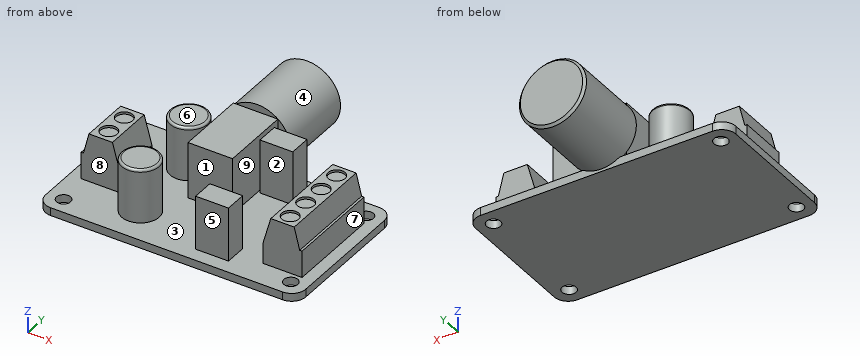
Autodesk Inventor part; units mm, degrees
ref_plane "YZ Plane" through (0, 0, 0) normal (1, 0, 0) x (0, 1, 0)
ref_plane "XZ Plane" through (0, 0, 0) normal (0, 1, 0) x (-1, 0, 0)
ref_plane "XY Plane" through (0, 0, 0) normal (0, 0, 1) x (1, 0, 0)
sketch "Board" plane through (0, 0, 0) normal (0, 0, 1) x (1, 0, 0)
  line L0 (-27.75, 16) -> (27.75, 16)
  line L1 (27.75, 16) -> (27.75, -16)
  line L2 (27.75, -16) -> (-27.75, -16)
  line L3 (-27.75, -16) -> (-27.75, 16)
  line L4 (-27.75, 16) -> (27.75, -16) construction
  line L5 (27.75, 16) -> (-27.75, -16) construction
  line L6 (-24.25, -12.5) -> (24.25, -12.5) construction
  line L7 (24.25, -12.5) -> (24.25, 12.5) construction
  line L8 (24.25, 12.5) -> (-24.25, 12.5) construction
  line L9 (-24.25, 12.5) -> (-24.25, -12.5) construction
  line L10 (-24.25, -12.5) -> (24.25, 12.5) construction
  line L11 (24.25, -12.5) -> (-24.25, 12.5) construction
  circle A0 centre (24.25, 12.5) radius 1.5
  circle A1 centre (-24.25, 12.5) radius 1.5
  circle A2 centre (24.25, -12.5) radius 1.5
  circle A3 centre (-24.25, -12.5) radius 1.5
  line L12 (-25.75, -14) -> (-22.75, -14) construction
  line L13 (-22.75, -14) -> (-22.75, -11) construction
  line L14 (-22.75, -11) -> (-25.75, -11) construction
  line L15 (-25.75, -11) -> (-25.75, -14) construction
  line L16 (-25.75, -14) -> (-22.75, -11) construction
  line L17 (-22.75, -14) -> (-25.75, -11) construction
  point P0 (0, 0)
  dimension "d0" = 55.5
  dimension "d1" = 32
  dimension "d2" = 3
  dimension "d3" = 2
  dimension "d5" = 2
  dimension "d6" = 48.5
extrude "BoardFeature" add sketch "Board" along normal blind 1.7
fillet "BoardFilletsFeature" radius 3 4 edges at (-27.75, 16, 0.85) (27.75, 16, 0.85) (-27.75, -16, 0.85) (27.75, -16, 0.85)
sketch "PotentiometerHousing" plane through (0, 0, 1.7) normal (0, 0, 1) x (1, 0, 0)
  line L0 (-5.75, 15) -> (3.75, 15)
  line L1 (3.75, 15) -> (3.75, 0)
  line L2 (3.75, 0) -> (-5.75, 0)
  line L3 (-5.75, 0) -> (-5.75, 15)
  line L4 (24.75, 16) -> (-24.75, 16)
  line L5 (-27.75, 13) -> (-27.75, -13)
  point P0 (0, 0)
  dimension "d10" = 1
  dimension "d11" = 22
  dimension "d12" = 15
  dimension "d13" = 9.5
extrude "PotentiometerHousingFeature" add sketch "PotentiometerHousing" along normal blind 12
sketch "IJ63" plane through (0, 0, 1.7) normal (0, 0, 1) x (1, 0, 0)
  line L0 (4.25, 13) -> (11.25, 13)
  line L1 (11.25, 13) -> (11.25, 8.3)
  line L2 (11.25, 8.3) -> (4.25, 8.3)
  line L3 (4.25, 8.3) -> (4.25, 13)
  line L4 (3.75, 15) -> (-5.75, 15)
  line L5 (3.75, 0) -> (3.75, 15)
  line L6 (-38.85, 0) -> (38.85, 0) construction
  line L7 (4.25, -13) -> (11.25, -13)
  line L8 (11.25, -13) -> (11.25, -8.3)
  line L9 (11.25, -8.3) -> (4.25, -8.3)
  line L10 (4.25, -8.3) -> (4.25, -13)
  point P0 (0, 0)
  dimension "d16" = 2
  dimension "d17" = 4.7
  dimension "d18" = 7
  dimension "d19" = 0.5
extrude "IJ63Feature" add sketch "IJ63" along normal blind 11.5
sketch "Capacitors" plane through (0, 0, 1.7) normal (0, 0, 1) x (1, 0, 0)
  line L0 (-38.85, 0) -> (38.85, 0) construction
  circle A0 centre (-10.75, 8) radius 4
  line L1 (0, -22.4) -> (0, 22.4) construction
  line L2 (-5.75, 15) -> (-5.75, 0)
  line L3 (24.75, 16) -> (-24.75, 16)
  circle A1 centre (-10.75, -8) radius 4
  point P0 (0, 0)
  dimension "d22" = 8
  dimension "d23" = 5
  dimension "d24" = 8
extrude "CapacitorsFeature" add sketch "Capacitors" along normal blind 11.5
sketch "TerminalBlocks" plane through (0, 0, 1.7) normal (0, 0, 1) x (1, 0, 0)
  line L0 (-38.85, 0) -> (38.85, 0) construction
  line L1 (25.18, 10.25) -> (16.83, 10.25)
  line L2 (16.83, 10.25) -> (16.83, -10.25)
  line L3 (16.83, -10.25) -> (25.18, -10.25)
  line L4 (25.18, -10.25) -> (25.18, 10.25)
  line L5 (-25.18, 5.25) -> (-16.83, 5.25)
  line L6 (-16.83, 5.25) -> (-16.83, -5.25)
  line L7 (-16.83, -5.25) -> (-25.18, -5.25)
  line L8 (-25.18, -5.25) -> (-25.18, 5.25)
  line L9 (27.75, -13) -> (27.75, 13)
  line L10 (-27.75, 13) -> (-27.75, -13)
  point P0 (0, 0)
  point P1 (25.18, 0)
  point P2 (-16.83, 0)
  dimension "d27" = 8.35
  dimension "d28" = 20.5
  dimension "d29" = 10.5
  dimension "d30" = 2.57
  dimension "d31" = 2.57
extrude "TerminalBlocksFeature" add sketch "TerminalBlocks" along normal blind 10.33
sketch "TerminalBlockProfiles" plane through (16.83, -10.25, 1.7) normal (0, -1, 0) x (1, 0, 0)
  line L0 (8.35, 0) -> (0, 0)
  line L1 (8.35, 0) -> (8.35, 10.33)
  line L2 (0, 10.33) -> (8.35, 10.33)
  line L3 (0, 0) -> (0, 10.33)
  line L4 (-33.66, 0) -> (-42.01, 0)
  line L5 (-33.66, 0) -> (-33.66, 10.33)
  line L6 (-42.01, 10.33) -> (-33.66, 10.33)
  line L7 (-42.01, 0) -> (-42.01, 10.33)
  line L8 (0, 10.33) -> (8.35, 10.33)
  line L9 (1.675, 10.33) -> (0, 4.33)
  line L10 (6.675, 10.33) -> (7.85, 5.72)
  line L11 (7.85, 5.72) -> (8.35, 5.72)
  line L12 (8.35, 0) -> (8.35, 10.33)
  line L13 (-16.83, -4.44) -> (-16.83, 14.74) construction
  line L14 (-35.335, 10.33) -> (-33.66, 4.33)
  line L15 (-40.335, 10.33) -> (-41.51, 5.72)
  line L16 (-41.51, 5.72) -> (-42.01, 5.72)
  line L17 (1.675, 10.33) -> (6.675, 10.33)
  point P0 (-16.83, -1.7)
  point P1 (4.175, 10.33)
  point P2 (6.675, 10.33)
  point P3 (1.675, 10.33)
  point P4 (-33.66, 4.33)
  dimension "d34" = 5
  dimension "d35" = 0.5
  dimension "d36" = 4.33
  dimension "d37" = 5.72
extrude "TerminalBlockProfilesFeature" cut sketch "TerminalBlockProfiles" against normal through all contours L11 L10 L2 L1 | L3 L2 L9 | L14 L6 L5 | L7 L6 L15 L16
sketch "TerminalBlockScrews" plane through (0, 0, 12.03) normal (0, 0, 1) x (1, 0, 0)
  line L0 (18.505, 10.25) -> (18.505, -10.25)
  line L1 (18.505, -10.25) -> (23.505, -10.25)
  line L2 (23.505, -10.25) -> (23.505, 10.25)
  line L3 (23.505, 10.25) -> (18.505, 10.25)
  line L4 (-18.505, -5.25) -> (-18.505, 5.25)
  line L5 (-18.505, 5.25) -> (-23.505, 5.25)
  line L6 (-23.505, 5.25) -> (-23.505, -5.25)
  line L7 (-23.505, -5.25) -> (-18.505, -5.25)
  line L8 (18.505, 0) -> (23.505, 0) construction
  line L9 (18.505, 0) -> (23.505, 10.25) construction
  line L10 (21.005, 5.125) -> (23.505, 5.125) construction
  line L11 (23.505, 5.125) -> (18.505, 10.25) construction
  circle A0 centre (21.005, 7.6875) radius 1.8
  circle A1 centre (21.005, 2.5625) radius 1.8
  circle A2 centre (21.005, -7.6875) radius 1.8
  line L12 (21.005, 7.6875) -> (21.005, -7.6875) construction
  circle A3 centre (21.005, -2.5625) radius 1.8
  line L13 (0, -22.4) -> (0, 22.4) construction
  circle A4 centre (-21.005, 2.5625) radius 1.8
  circle A5 centre (-21.005, -2.5625) radius 1.8
  point P0 (0, 0)
  dimension "d41" = 3.6
  dimension "d42" = 2.5625
  dimension "d43" = 2.5625
extrude "TerminalBlockScrewsFeature" cut sketch "TerminalBlockScrews" against normal blind 0.5 contours A0 | A1 | A2 | A3 | A4 | A5
fillet "FilletsFeature" radius 0.5 2 edges at (-14.75, -8, 13.2) (-14.75, 8, 13.2)
sketch "PotentiometerShaft" plane through (-5.75, 15, 1.7) normal (0, 1, 0) x (1, 0, 0)
  line L0 (0, 0) -> (9.5, 0)
  line L1 (0, 0) -> (0, -12)
  line L2 (9.5, -12) -> (0, -12)
  line L3 (9.5, 0) -> (9.5, -12)
  line L4 (9.5, -12) -> (0, 0) construction
  circle A0 centre (4.75, -6) radius 3
  point P0 (5.75, 1.7)
  dimension "d48" = 6
extrude "PotentiometerShaftFeature" add sketch "PotentiometerShaft" along normal blind 0.5 contours A0
sketch "PotentiometerKnob" plane through (-1, 15.5, 7.7) normal (0, 1, 0) x (1, 0, 0)
  circle A0 centre (0, 0) radius 3
  circle A1 centre (0, 0) radius 3
  circle A2 centre (0, 0) radius 7.15
  point P0 (1, 7.7)
  dimension "d51" = 14.3
extrude "PotentiometerKnobFeature" add sketch "PotentiometerKnob" along normal blind 17 contours A0 | A2
chamfer "PotentiometerKnobChamferFeature" distance 0.5 angle 45 1 edges at (-8.15, 32.5, 7.7)
equation "\"d5\" = d3"
equation "\"d31\" = d30"
equation "\"d43\" = d42"
properties part number "LQ-AMP10W"
Design review of the part built by this model. Coordinates are the model's own, in mm. Face numbers are marked on the shaded views. A direction names the side the tool comes from. Give positions to 0.01 mm unless a question says otherwise; leave off trailing zeros. Write each loop counter-clockwise with the first axis right and the second up, starting at its lowest first coordinate (ties: lowest second). Pieces come first, ordered by that corner, then holes. Notation, with made-up numbers: M 47,-36 L 65,-36 A24 cw 65,-1 Z; hole C -24.5,-14.5 d7. An arc over 180 degrees is marked long. Answer as a JSON object with one key per item and string values. Group by question number.
1) We need section B-B (y = 21). Give the boundary of the cut face in (x, z).
2) Mouldability with a two-part tool opening along Y and no side actions: class the marked faces 1, 2, 3 and 4 as released by +Y, released by -Y, zero draft, split by the parting line, or undercut.
3) We need section A-A (x = 7). Give the boundary of the cut face in (y, z).
4) We need section C-C (x = 13.5). Give the boundary of the cut face in (y, z).
5) Clearance check with flat-ended pins moving along their axes: pin 1 Ø2.5 at (x, z) = (21, 9) entering from -Y; pin 2 Ø4 at (x, y) = (-21, -2.56) entering from +Z; pin 3 Ø8 at (x, y) = (-16.5, 4.5) entering from +Z; pin 4 Ø1.8 at (x, y) = (-24.25, -12.5) entering from +Z. State where each tip first meets the part, or that it passes through.
6) For line 1 along Y through (x, z) = (8, 5.5); line 2 along Y through (x, z) = (5, 1.25); line 3 along X through (y, z) = (4.5, 8.5), list the stretches that pass through material, from the lowest coordinate up.
7) Tool access review of the marked faces 5, 6, 7, 8 and 9: name each direction out of +Z, -Z, +X, -X, +Y, -Y from which nothing blocks a thin tool from reaching the whole face with its end or side.
Answer key:
{
 "1": {"outline": "C -1,7.7 d14.3"},
 "2": {"face 1": "released by -Y", "face 2": "undercut", "face 3": "undercut", "face 4": "zero draft"},
 "3": {"outline": "M -16,0 L 16,0 L 16,1.7 L 13,1.7 L 13,13.2 L 8.3,13.2 L 8.3,1.7 L -8.3,1.7 L -8.3,13.2 L -13,13.2 L -13,1.7 L -16,1.7 Z"},
 "4": {"outline": "M -16,0 L 16,0 L 16,1.7 L -16,1.7 Z"},
 "5": {"pin 1": "stops at y = -10.25", "pin 2": "stops at z = 12.03", "pin 3": "stops at z = 13.2", "pin 4": "passes through"},
 "6": {"line 1": "y = -13 to -8.3, 8.3 to 13", "line 2": "y = -16 to 16", "line 3": "x = -24.4 to -17.52, -12.69 to -8.81, -5.75 to 3.75, 17.52 to 24.4"},
 "7": {"face 5": "+Z, +X, -X, -Y", "face 6": "+Z, -X, +Y, -Y", "face 7": "+Z, +X, +Y, -Y", "face 8": "+Z, -X, -Y", "face 9": "+Z, -Y"}
}
